Build history of the part. All positions in model axes, mm. A direction names the side the tool comes from. Round coordinates to 2 decimals unless told otherwise and drop trailing zeros. Write each loop counter-clockwise with the first axis right and the second up, starting at its lowest first coordinate (ties: lowest second). Pieces come first, ordered by that corner, then holes.
Item 1: Drop flat-ended pins along their axis: pin 1 Ø1.8 at (x, z) = (34, 10.5) entering from -Y; pin 2 Ø1 at (x, y) = (8, -3.5) entering from +Z; pin 3 Ø1.1 at (x, z) = (12.5, -1.5) entering from -Y. Give the stop position or say it passes through.
Item 2: Band-saw the part on A-A, the plane y = 2.75. Count the separate pieces of the cut face and the enclosed holes in it, then the cut area to 3 significant figures.
Item 3: Band-saw the part on B-B, the plane x = -25. Write the cut outline in (y, z), then the cut area to 3 significant figures.
Item 4: 3-axis set-ups, long thin cutter, end or side, ignore diameter. For faces 1 (the flat face through (-11, 1, -3)), 2 (the flat face through (-8.42, -0.77, 8.57)), 3 (the flat face through (-11.6, -1.66, -3.11)): which of +Z, -Z, +X, -X, +Y, -Y reach the whole face in a straight line?
Item 5: Band-saw the part on C-C, the plane z = 0. Write the cut outline in (x, y).
Item 6: Mould opens along Z. For faces 4 (the flat face through (10, -2.5, 6)), 5 (the cylindrical face through (-34.605, 2.067, -21.946)), 6 (the cylindrical face through (39, 0, 0)) say: +Z half, -Z half, draft (parallel to the pull), parting line (faces both ways), or undercut.
Item 7: Wall check: probe 1 along Z at (x, y) = (-34, -1.25); probe 2 along Z at (x, y) = (34, -1.75); probe 3 along X at (y, z) = (0, 7.5). Give the ranges that are in metal, low to high.
Item 8: Band-saw the part on D-D, the plane x = 34. Write the cut outline in (y, z).
```python
from build123d import *
from build123d.topology import SkipClean

# Parameters (mm, degrees)
EXTRUDE_1_DEPTH                  = 4
SKETCH_9_R                       = 13.4
CUT_EXTRUDE_1_DEPTH              = 46.730186967
FILLET_4_R                       = 3
CHAMFER_3_SIZE                   = 5
SKETCH_10_R                      = 3.9
EXTRUDE_8_DEPTH                  = 1
PATTERN_CIRCULAR_4_COUNT         = 4
EXTRUDE_START                    = -3.5
EXTRUDE_9_DEPTH                  = 3.5
CUT_EXTRUDE_2_DEPTH              = 1.7
FILLET_5_R                       = 0.5
PATTERN_CIRCULAR_5_COUNT         = 4
FILLET_5_OF_PATTERN_CIRCULAR_5_R = 0.5


with BuildPart() as part:
    # ｽｹｯﾁ2 → ﾎﾞｽ - 押し出し1 (new, symmetric)
    with BuildSketch(Plane(origin=(0, 0, 0), x_dir=(1, 0, 0), z_dir=(0, 1, 0))):
        with BuildLine():
            Line((-35, 22.5), (35, 22.5))
            ThreePointArc((35, 22.5), (39, 0), (35, -22.5))
            Line((35, -22.5), (-35, -22.5))
            ThreePointArc((-35, -22.5), (-39, 0), (-35, 22.5))
        make_face()
    extrude(amount=EXTRUDE_1_DEPTH, both=True)

    # ｽｹｯﾁ9 → ｶｯﾄ - 押し出し1 (cut, through all)
    with BuildSketch(Plane.XZ.offset(4)):
        with Locations(Location((0, 0, 0), (0, 0, 270))):
            Circle(SKETCH_9_R)
    extrude(amount=-CUT_EXTRUDE_1_DEPTH, mode=Mode.SUBTRACT)

    # ﾌｨﾚｯﾄ4
    fillet_4_edges = [part.edges().sort_by_distance(p)[0] for p in [
        (-35, 0, -22.5),
        (35, 0, -22.5),
        (35, 0, 22.5),
        (-35, 0, 22.5),
    ]]
    fillet(fillet_4_edges, radius=FILLET_4_R)

    # 面取り3
    # the kernel refuses this chamfer: 5 mm, written as the material it takes off along each edge
    with BuildSketch(Plane(origin=(-45.727009416, -4, -22.5), x_dir=(0, -0.027495876610586317, 0.9996219169112968), z_dir=(1, 0, 0))) as chamfer_3_piece_1:
        Polygon((CHAMFER_3_SIZE * 0.999621916911, -CHAMFER_3_SIZE * 0.0274958766106), (-CHAMFER_3_SIZE * 0.0274958766106, -CHAMFER_3_SIZE * 0.999621916911), (0, 0), align=None)
    extrude(amount=91.454018832, mode=Mode.SUBTRACT)
    with BuildSketch(Plane(origin=(45.727009416, -4, 22.5), x_dir=(0, 0.9996219169112968, 0.027495876610586317), z_dir=(-1, 0, 0))) as chamfer_3_piece_2:
        Polygon((CHAMFER_3_SIZE * 0.999621916911, CHAMFER_3_SIZE * 0.0274958766106), (-CHAMFER_3_SIZE * 0.0274958766106, CHAMFER_3_SIZE * 0.999621916911), (0, 0), align=None)
    extrude(amount=91.454018832, mode=Mode.SUBTRACT)

    # ｽｹｯﾁ10 → ﾎﾞｽ - 押し出し8 (add)
    with BuildSketch(Plane.XZ.offset(4)):
        with Locations(Location((-23.5, 0, 0), (0, 0, 90))):
            Circle(SKETCH_10_R)
    extrude_8 = extrude(amount=EXTRUDE_8_DEPTH)

    # ｽｹｯﾁ12 → M2 ねじ穴1 (revolve, cut)
    with BuildSketch(Plane(origin=(-13, -4, 10.5), x_dir=(0, 0, -1), z_dir=(1, 0, 0))):
        Polygon((0, 0), (0, 10.480688495), (0.8, 10), (0.8, 0), align=None)
    hole_wizard_m2_1 = revolve(axis=Axis((-13, -10.35, 10.5), (0, 1, 0)), mode=Mode.SUBTRACT)

    # 円形ﾊﾟﾀｰﾝ4: M2 ねじ穴1 ×4 about axis
    pattern_circular_4_axis = Axis((-23.5, 0, 0), (0, 1, 0))
    for i in range(1, PATTERN_CIRCULAR_4_COUNT):
        add(hole_wizard_m2_1.rotate(pattern_circular_4_axis, i * 360 / PATTERN_CIRCULAR_4_COUNT), mode=Mode.SUBTRACT)

    # ﾐﾗｰ3: ﾎﾞｽ - 押し出し8, M2 ねじ穴1 across plane
    add(extrude_8.mirror(Plane(origin=(0, 0, 0), x_dir=(0, 0, 1), z_dir=(1, 0, 0))))
    add(hole_wizard_m2_1.mirror(Plane(origin=(0, 0, 0), x_dir=(0, 0, 1), z_dir=(1, 0, 0))), mode=Mode.SUBTRACT)

    # ﾐﾗｰ3 copy 1 sketch → ﾐﾗｰ3 copy 1 (revolve, cut)
    with BuildSketch(Plane(origin=(13, -4, -10.5), x_dir=(1, 0, 0), z_dir=(0, 0, -1))):
        Polygon((0, 0), (0, -10.480688495), (0.8, -10), (0.8, 0), align=None)
    revolve(axis=Axis((13, -10.35, -10.5), (0, -1, 0)), mode=Mode.SUBTRACT)

    # ﾐﾗｰ3 copy 2 sketch → ﾐﾗｰ3 copy 2 (revolve, cut)
    with BuildSketch(Plane(origin=(34, -4, -10.5), x_dir=(0, 0, 1), z_dir=(1, 0, 0))):
        Polygon((0, 0), (0, -10.480688495), (0.8, -10), (0.8, 0), align=None)
    revolve(axis=Axis((34, -10.35, -10.5), (0, -1, 0)), mode=Mode.SUBTRACT)

    # ﾐﾗｰ3 copy 3 sketch → ﾐﾗｰ3 copy 3 (revolve, cut)
    with BuildSketch(Plane(origin=(34, -4, 10.5), x_dir=(-1, 0, 0), z_dir=(0, 0, 1))):
        Polygon((0, 0), (0, -10.480688495), (0.8, -10), (0.8, 0), align=None)
    revolve(axis=Axis((34, -10.35, 10.5), (0, -1, 0)), mode=Mode.SUBTRACT)

    # ｽｹｯﾁ13 → ﾎﾞｽ - 押し出し9 (add)
    with BuildSketch(Plane(origin=(0, 1, 0), x_dir=(1, 0, 0), z_dir=(0, 1, 0)).offset(EXTRUDE_START)):
        with BuildLine():
            Line((-9.392184142, -9.557556019), (-7.079183569, -7.203829536))
            ThreePointArc((-7.079183569, -7.203829536), (-2.571479677, -9.767163983), (2.614072356, -9.755850846))
            Line((2.614072356, -9.755850846), (3.468175204, -12.943406072))
            ThreePointArc((3.468175204, -12.943406072), (-3.411666106, -12.958415581), (-9.392184142, -9.557556019))
        make_face()
    extrude_9 = extrude(amount=EXTRUDE_9_DEPTH)

    # ｽｹｯﾁ14 → ｶｯﾄ - 押し出し2 (cut)
    with BuildSketch(Plane.XZ.offset(2.5)):
        with BuildLine():
            Line((0, 0), (3.468175204, 12.943406072))
            ThreePointArc((3.468175204, 12.943406072), (0, 13.4), (-3.468175204, 12.943406072))
            Line((-3.468175204, 12.943406072), (0, 0))
        make_face()
    cut_extrude_2 = extrude(amount=-CUT_EXTRUDE_2_DEPTH, mode=Mode.SUBTRACT)

    # ﾌｨﾚｯﾄ5
    fillet_5_edges = [part.edges().sort_by_distance(p)[0] for p in [
        (-7.079183569, -0.75, 7.203829536),
        (2.614072356, 0.1, 9.755850846),
        (-2.614072356, -1.65, 9.755850846),
    ]]
    fillet(fillet_5_edges, radius=FILLET_5_R)

    # 円形ﾊﾟﾀｰﾝ5: ﾎﾞｽ - 押し出し9, ｶｯﾄ - 押し出し2 ×4 about axis
    with SkipClean():  # the faces are left unmerged after this step: merging them gives an invalid solid
        pattern_circular_5_axis = Axis((0, 0, 0), (0, 1, 0))
        add([extrude_9.rotate(pattern_circular_5_axis, i * 360 / PATTERN_CIRCULAR_5_COUNT) for i in range(1, PATTERN_CIRCULAR_5_COUNT)])
        add([cut_extrude_2.rotate(pattern_circular_5_axis, i * 360 / PATTERN_CIRCULAR_5_COUNT) for i in range(1, PATTERN_CIRCULAR_5_COUNT)], mode=Mode.SUBTRACT)

    # ﾌｨﾚｯﾄ5 of 円形ﾊﾟﾀｰﾝ5
    fillet_5_of_pattern_circular_5_edges = [part.edges().sort_by_distance(p)[0] for p in [
        (7.203829536, -0.75, 7.079183569),
        (9.755850846, 0.1, -2.614072356),
        (9.755850846, -1.65, 2.614072356),
        (7.079183569, -0.75, -7.203829536),
        (-2.614072356, 0.1, -9.755850846),
        (2.614072356, -1.65, -9.755850846),
        (-7.203829536, -0.75, -7.079183569),
        (-9.755850846, 0.1, 2.614072356),
        (-9.755850846, -1.65, -2.614072356),
    ]]
    fillet(fillet_5_of_pattern_circular_5_edges, radius=FILLET_5_OF_PATTERN_CIRCULAR_5_R)


solid = part.part
```
Results:
1. pin 1: stops at y = -4
1. pin 2: stops at z = 18.5
1. pin 3: stops at y = -0.8
2. separate pieces: 1
2. enclosed holes: 9
2. area: 2,810 mm2
3. outline: (-5, -3.6) - (-4, -3.6) - (-4, -17.5) - (1, -22.5) - (4, -22.5) - (4, 22.5) - (1, 22.5) - (-4, 17.5) - (-4, 3.6) - (-5, 3.6) - close
3. area: 342 mm2
4. face 1: +Y
4. face 2: +Y, -Y
4. face 3: -Y
5. outline: (-39, -4) - (-27.4, -4) - (-27.4, -5) - (-19.6, -5) - (-19.6, -4) - (-13.4, -4) - (-13.4, -0.8) - (-10.1, -0.8) - (-10.1, 1) - (-13.4, 1) - (-13.4, 4) - (-39, 4) - close; (10.1, -0.8) - (13.4, -0.8) - (13.4, -4) - (19.6, -4) - (19.6, -5) - (27.4, -5) - (27.4, -4) - (39, -4) - (39, 4) - (13.4, 4) - (13.4, 1) - (10.1, 1) - close
6. face 4: undercut
6. face 5: -Z half
6. face 6: parting line
7. probe 1: z = -20.25 to -11.3, -9.7 to 9.7, 11.3 to 20.25
7. probe 2: z = -19.75 to -11.3, -9.7 to 9.7, 11.3 to 19.75
7. probe 3: x = -38.57 to -11.1, -7.36 to -6.77, 7.63 to 38.57
8. outline: (-4, -17.5) - (0.78, -22.28) - (4, -22.28) - (4, -11.3) - (-4, -11.3) - close; (-4, -9.7) - (4, -9.7) - (4, 9.7) - (-4, 9.7) - close; (-4, 11.3) - (4, 11.3) - (4, 22.28) - (0.78, 22.28) - (-4, 17.5) - close
